The model under review builds one solid part; all positions refer to its coordinate system, in mm. Face numbers are marked on the shaded views. Coordinates: 2 decimals unless noted, no trailing zeros. Order: outer loops, then holes, each group sorted by start corner. A loop starts at its lowest first (then second) coordinate and runs counter-clockwise, first axis right, second up. Notation, with made-up numbers: (83, 60) - (87, 60) arc R14 cw to (87, 80) - close; hole circle Ø7 at (55, -19.5). An arc over 180 degrees is marked (long way). Answer in a Markdown table with one row per item.
```python
from build123d import *

# Parameters (mm, degrees)
F1_DEPTH      = 31.75
F1_DEPTH_BACK = 12.7
F2_R          = 3.175
F3_DEPTH      = 25.4
F4_R          = 1.5875
F5_DEPTH      = 25.4
F7_DEPTH      = 25.4
F8_R          = 5.08
F9_SIZE       = 0.508


with BuildPart() as f1:
    # F0 (on Front) → F1 (new body, two sides)
    with BuildSketch(Plane.XZ) as f1_sk:
        Polygon((-37.854384, 0), (0, 0), (37.854384, 0), (37.854384, 35.133872), (19.893872, 53.094384), (0, 53.094384), (-19.893872, 53.094384), (-37.854384, 35.133872), align=None)
    extrude(amount=F1_DEPTH)
    extrude(f1_sk.sketch, amount=-F1_DEPTH_BACK)

    # F2 (on face) → F3 (cut)
    with BuildSketch(Plane(origin=(-36.494128, 0, 36.494128), x_dir=(0, -1, 0), z_dir=(-0.707107, 0, 0.707107))):
        with Locations((0, 10.776307)):
            Circle(F2_R)
    extrude(amount=-F3_DEPTH, mode=Mode.SUBTRACT)

    # F4 (on face) → F5 (cut)
    with BuildSketch(Plane(origin=(36.494128, 0, 36.494128), x_dir=(0.707107, 0, -0.707107), z_dir=(0.707107, 0, 0.707107))):
        with Locations((-10.776307, 0)):
            Circle(F4_R)
    extrude(amount=-F5_DEPTH, mode=Mode.SUBTRACT)

    # F6 (on face) → F7 (cut)
    with BuildSketch(Plane.XZ.offset(31.75)):
        with BuildLine():
            Line((0, 24.220256), (-4.490128, 19.730128))
            ThreePointArc((-4.490128, 19.730128), (0, 8.89), (4.490128, 19.730128))
            Line((4.490128, 19.730128), (0, 24.220256))
        make_face()
    extrude(amount=-F7_DEPTH, mode=Mode.SUBTRACT)

    # F8
    f8_edges = [f1.edges().sort_by_distance(p)[0] for p in [
        (-37.854384, 12.7, 17.566936),
        (-28.874128, 12.7, 44.114128),
        (0, 12.7, 53.094384),
        (28.874128, 12.7, 44.114128),
        (37.854384, 12.7, 17.566936),
        (-19.893872, -9.525, 53.094384),
        (-37.854384, -9.525, 35.133872),
        (-28.874128, -31.75, 44.114128),
        (-37.854384, -31.75, 17.566936),
        (0, -31.75, 53.094384),
        (19.893872, -9.525, 53.094384),
        (28.874128, -31.75, 44.114128),
        (37.854384, -31.75, 17.566936),
        (37.854384, -9.525, 35.133872),
    ]]
    fillet(f8_edges, radius=F8_R)

    # F9
    f9_edges = [f1.edges().sort_by_distance(p)[0] for p in [
        (0, -6.35, 8.89),
        (-10.913616, 3.175, 26.153616),
        (9.791084, 0, 27.276148),
    ]]
    chamfer(f9_edges, length=F9_SIZE)


solid = f1.part
```
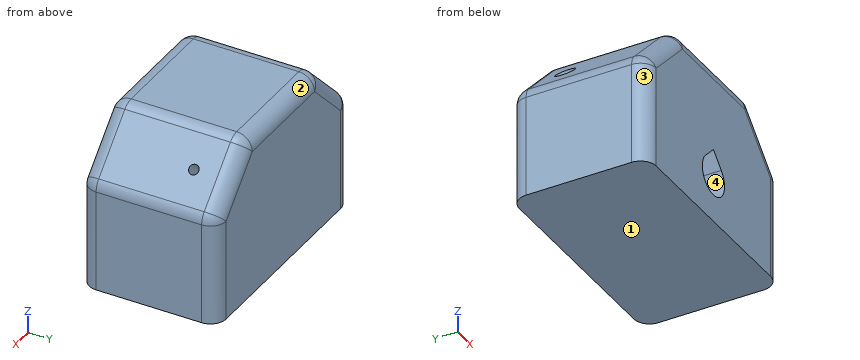
Item 1: We need section A-A, the plane z = 15.24. Write out the cut boundary in (x, y).
Check values:
| item | result |
|---|---|
| outline | (-37.85, -26.67) arc R5.08 ccw to (-32.77, -31.75) - (-6.35, -31.75) - (-6.35, -6.86) - (-5.84, -6.35) - (5.84, -6.35) - (6.35, -6.86) - (6.35, -31.75) - (32.77, -31.75) arc R5.08 ccw to (37.85, -26.67) - (37.85, 7.62) arc R5.08 ccw to (32.77, 12.7) - (-32.77, 12.7) arc R5.08 ccw to (-37.85, 7.62) - close |
Item 2: Clearance check with a flat-ended pin moving along its axis: pin 1 Ø1.5 at (y, z) = (5.5, 35.5) entering from -X. State where the tip first meets the part, or that it passes through.
Check values:
| item | result |
|---|---|
| pin 1 | x = -37.55 |
Item 3: We need section B-B, the plane z = 39. State how many separate pieces and enclosed holes the cut face has, then the cut area to 3 significant figures.
Check values:
| item | result |
|---|---|
| separate pieces | 1 |
| enclosed holes | 2 |
| area | 2,930 mm^2 |
Item 4: Mouldability with a two-part tool opening along Z and no side actions: class the marked faces 1, 2, 3 and 4 as +Z half, -Z half, draft (parallel to the pull), parting line (faces both ways), or undercut.
Check values:
| item | result |
|---|---|
| face 1 | -Z half |
| face 2 | +Z half |
| face 3 | draft |
| face 4 | undercut |
Item 5: To check wall thickness, follow line 1 (X direction, y = -25, z = 15); line 2 (X direction, y = -27, z = 8.5); line 3 (X direction, y = -22.5, z = 14). State the ranges of each line that lie inside material, in increasing order. Write a range as from..to.
Check values:
| item | result |
|---|---|
| line 1 | -37.85..-6.35, 6.35..37.85 |
| line 2 | -37.84..37.84 |
| line 3 | -37.85..-6.23, 6.23..37.85 |
Item 6: We need section C-C, the plane z = 21. Write out the cut boundary in (x, y).
Check values:
| item | result |
|---|---|
| outline | (-37.85, -26.67) arc R5.08 ccw to (-32.77, -31.75) - (-3.22, -31.75) - (-3.22, -6.86) - (-2.5, -6.35) - (2.5, -6.35) - (3.22, -6.86) - (3.22, -31.75) - (32.77, -31.75) arc R5.08 ccw to (37.85, -26.67) - (37.85, 7.62) arc R5.08 ccw to (32.77, 12.7) - (-32.77, 12.7) arc R5.08 ccw to (-37.85, 7.62) - close |
